```python
from build123d import *

# Parameters (mm, degrees)
SKETCH1_W           = 38.1
SKETCH1_H           = 30.48
BOSS_EXTRUDE1_DEPTH = 10.16
SKETCH3_R           = 1.65
CUT_EXTRUDE1_DEPTH  = 10


with BuildPart() as part:
    # Sketch1 → Boss-Extrude1 (new body)
    with BuildSketch(Plane(origin=(0, 0, 0), x_dir=(1, 0, 0), z_dir=(0, 1, 0))):
        Rectangle(SKETCH1_W, SKETCH1_H)
    extrude(amount=BOSS_EXTRUDE1_DEPTH)

    # Sketch3 → Cut-Extrude1 (cut)
    with BuildSketch(Plane.XZ):
        with Locations(Location((0, 7.62, 0), (0, 0, 270))):
            Circle(SKETCH3_R)
        with Locations(Location((0, -7.62, 0), (0, 0, 270))):
            Circle(SKETCH3_R)
    extrude(amount=-CUT_EXTRUDE1_DEPTH, mode=Mode.SUBTRACT)


solid = part.part
```
CAD build for the part. Positions are in the model's coordinates, mm. A direction names the side the tool comes from. Give positions to 0.01 mm unless a question says otherwise; leave off trailing zeros. Order: outer loops, then holes, each group sorted by start corner. A loop starts at its lowest first (then second) coordinate and runs counter-clockwise, first axis right, second up.
(1) Tool access for faces 5 (the flat face through (0, 0, 0)), 6 (the cylindrical face through (0.07, 4.93, 9.27)): list every direction of +Z, -Z, +X, -X, +Y, -Y with a clear straight run to the whole face (end or side of a thin tool).
(2) Mould opens along Z. For faces 1 (the cylindrical face through (-1, 4.93, -6.31)), 2 (the flat face through (0, 5, 15.24)), 3 (the flat face through (19.05, 5, 0)), 4 (the flat face through (0, 10, 8)) say: released by +Z, released by -Z, zero draft, split by the parting line, or undercut.
(3) Drill centre lines: L1, parallel to X at y = 4, z = -7.62; L2, parallel to Z at x = 0.5, y = 6.5; L3, parallel to Y at x = 1, z = 6.5. Where is each one in solid material? Low to high.
(4) Saw through at B-B, the plane x = 0. Give the cut face in (y, z), then the cut area to 3 significant figures.
(5) Flat gauge pins, fed straight in: pin 1 (2.5 mm diameter, centred on x = -0.5, z = -8, fed in from -Y); pin 2 (2 mm diameter, centred on x = 0, z = -7.62, fed in from -Y). Where does each tip first touch, or does it go through?
(6) Saw through at A-A, the plane z = 7.62. Give the cut face in (x, y), then the cut area to 3 significant figures.
Results found:
1. face 5: +Z, -Z, +X, -X, -Y
1. face 6: -Y
2. face 1: undercut
2. face 2: released by +Z
2. face 3: zero draft
2. face 4: undercut
3. L1: x = -19.05 to -1.65, 1.65 to 19.05
3. L2: z = -15.24 to -9.19, -6.05 to 6.05, 9.19 to 15.24
3. L3: y = 10 to 10.16
4. outline: (0, -15.24) - (10.16, -15.24) - (10.16, 15.24) - (0, 15.24) - (0, 9.27) - (10, 9.27) - (10, 5.97) - (0, 5.97) - (0, -5.97) - (10, -5.97) - (10, -9.27) - (0, -9.27) - close
4. area: 244 mm2
5. pin 1: stops at y = 0
5. pin 2: stops at y = 10
6. outline: (-19.05, 0) - (-1.65, 0) - (-1.65, 10) - (1.65, 10) - (1.65, 0) - (19.05, 0) - (19.05, 10.16) - (-19.05, 10.16) - close
6. area: 354 mm2
